Source: three-view drawing plus pictorial views. Frame: mm from the lowest corner of the part. A direction names the side the tool comes from. Round coordinates to 2 decimals unless told otherwise and drop trailing zeros. Loops run counter-clockwise (first coordinate to the right, second up) from the corner with the lowest first, then second, coordinate; pieces in that order, holes last. Notation, with made-up numbers: (64.25, -34.5) -> (115.25, -34.5) arc R22 cw to (115.25, -2.5) -> close; hole circle Ø3 at (55.5, 72). An arc over 180 degrees is marked (long way). One line per question, with ' | ' between items. Start each with the question number.
Q1. Mould query, pull axis X, two halves, no side actions, for the marked faces 1, 2 and 3. Classes: pulls with the +X half, pulls with the -X half, needs draft (parallel to the pull), parting line crosses it, or undercut.
Q2. Cut plane A-A on x = 136. Return loops of the section in (y, z), and give its area (3 significant figures).
Q3. Access query for the marked faces 4, 5, 6, 7 and 8. Directions: +Z, -Z, +X, -X, +Y, -Y. A direction counts if a zero-diameter tool reaches every point of the face in a straight line with its end or side. Return the directions, or none.
Q4. Cut plane B-B on y = 27. Return loops of the section in (x, z), and give its area (3 significant figures).
Q5. Cut plane C-C on z = 38. Return loops of the section in (x, y), and give its area (3 significant figures).
Q6. Material intervals for L1, parallel to Z at x = 30, y = 31; L2, parallel to X at y = 28, z = 41; L3, parallel to Z at x = 136, y = 62, sorted ascending.
Q7. Cut plane D-D on y = 79.5. Return loops of the section in (x, z), and give its area (3 significant figures).
Q8. Contact query for flat-ended pins moving along their axis: P1, Ø5, axis at x = 99, z = 52, coming from the -Y side; P2, Ø6, axis at y = 8, z = 25.5, coming from the +X side; P3, Ø18.5, axis at x = 225, z = 46, coming from the +Y side; P4, Ø18, axis at x = 240, z = 41, coming from the +Y side. Output: stop coordinate, or through.
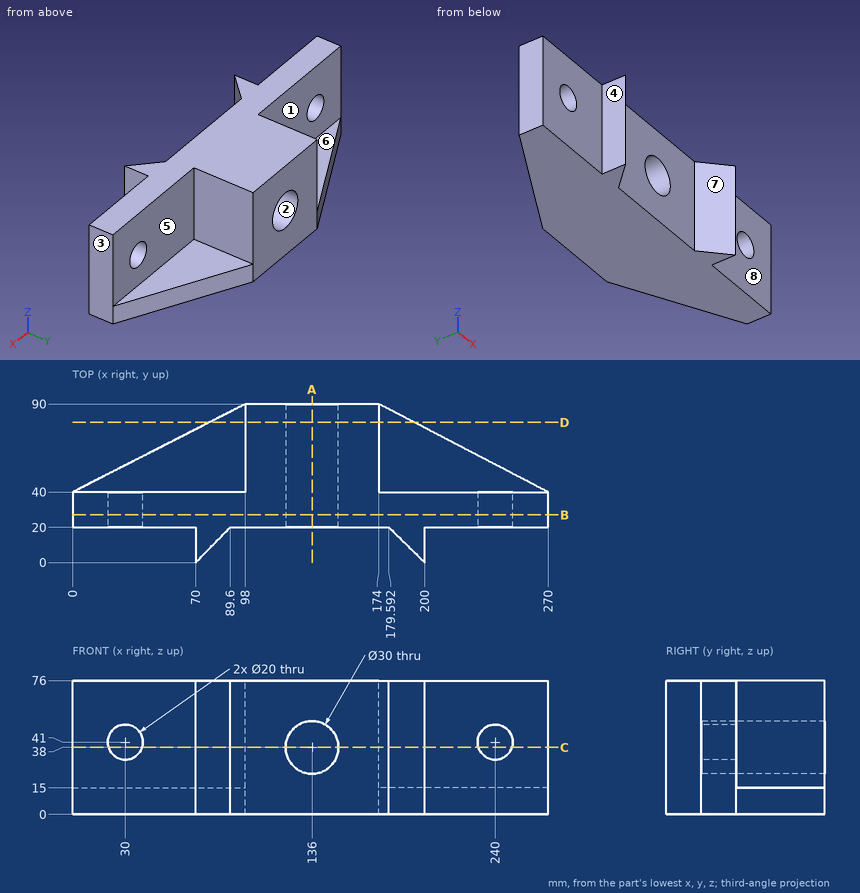
Results:
1) face 1: needs draft | face 2: undercut | face 3: pulls with the +X half
2) outline: (20, 0) -> (90, 0) -> (90, 23) -> (20, 23) -> close; (20, 53) -> (90, 53) -> (90, 76) -> (20, 76) -> close | area: 3,220 mm^2
3) face 4: +Z, -Z, -X, -Y | face 5: +Z, +X, +Y | face 6: +Z, -X, +Y | face 7: +Z, -Z, -Y | face 8: +Z, -Z, +X, -Y
4) outline: (0, 0) -> (270, 0) -> (270, 76) -> (0, 76) -> close; hole circle Ø20 at (30, 41); hole circle Ø30 at (136, 38); hole circle Ø20 at (240, 41) | area: 19,200 mm^2
5) outline: (0, 20) -> (20.46, 20) -> (20.46, 40) -> (0, 40) -> close; (39.54, 20) -> (70, 20) -> (70, 0) -> (89.6, 20) -> (121, 20) -> (121, 90) -> (98, 90) -> (98, 40) -> (39.54, 40) -> close; (151, 20) -> (179.59, 20) -> (200, 0) -> (200, 20) -> (230.46, 20) -> (230.46, 40) -> (174, 40) -> (174, 90) -> (151, 90) -> close; (249.54, 20) -> (270, 20) -> (270, 40) -> (249.54, 40) -> close | area: 6,740 mm^2
6) L1: 0 to 31, 51 to 76 | L2: 0 to 20, 40 to 121.3, 150.7 to 230, 250 to 270 | L3: 0 to 23, 53 to 76
7) outline: (77.42, 0) -> (194.16, 0) -> (194.16, 15) -> (174, 15) -> (174, 76) -> (98, 76) -> (98, 15) -> (77.42, 15) -> close; hole circle Ø30 at (136, 38) | area: 5,680 mm^2
8) P1: y = 20 | P2: x = 200 | P3: y = 40 | P4: through
